Autodesk Inventor part; units mm, degrees
ref_plane "YZ Plane" through (0, 0, 0) normal (1, 0, 0) x (0, 1, 0)
ref_plane "XZ Plane" through (0, 0, 0) normal (0, 1, 0) x (-1, 0, 0)
ref_plane "XY Plane" through (0, 0, 0) normal (0, 0, 1) x (1, 0, 0)
sketch "Boceto1" plane through (0, 0, 0) normal (0, 0, 1) x (1, 0, 0)
  line L0 (85, 15) -> (-82, 15)
  line L1 (-85, -15) -> (85, 15) construction
  line L2 (85, -15) -> (-85, 15) construction
  line L3 (-28, -15) -> (-28, 5)
  line L4 (28, 5) -> (28, -15)
  line L5 (-28, 5) -> (28, 5)
  line L6 (-82, -15) -> (-28, -15)
  line L7 (28, -15) -> (85, -15)
  line L8 (-82, -13.0321) -> (-82, -3.7)
  line L9 (-82, -3.7) -> (-85, -3.7)
  line L10 (-85, -13.0321) -> (-85, -3.7)
  line L11 (-82, -13.0321) -> (-85, -13.0321)
  line L12 (-82, 3.7) -> (-82, 13.0321)
  line L13 (-82, 13.0321) -> (-85, 13.0321)
  line L14 (-85, 3.7) -> (-85, 13.0321)
  line L15 (-82, 3.7) -> (-85, 3.7)
  line L16 (-82, -3.7) -> (-82, 3.7)
  line L17 (-82, 13.0321) -> (-82, 15)
  line L18 (-82, -15) -> (-82, -13.0321)
  line L19 (82, 15) -> (82, 11.3)
  line L20 (82, 11.3) -> (85, 11.3)
  line L21 (85, 15) -> (85, 11.3)
  line L22 (82, 15) -> (85, 15)
  line L23 (82, 3.7) -> (82, -3.7)
  line L24 (82, -3.7) -> (85, -3.7)
  line L25 (85, 3.7) -> (85, -3.7)
  line L26 (82, 3.7) -> (85, 3.7)
  line L27 (82, -11.3) -> (82, -15)
  line L28 (82, -15) -> (85, -15)
  line L29 (85, -11.3) -> (85, -15)
  line L30 (82, -11.3) -> (85, -11.3)
  line L31 (82, -3.7) -> (82, -11.3)
  line L32 (82, 11.3) -> (82, 3.7)
  point P0 (0, 0)
  point P1 (28, 0)
  dimension "d0" = 30
  dimension "d1" = 170
  dimension "d7" = 20
  dimension "d11" = 30
extrude "Extrusión1" add sketch "Boceto1" along normal blind 3
Part model, mm, in its own coordinate system. A direction names the side the tool comes from. Coordinates: 2 decimals unless noted, no trailing zeros. Write each loop counter-clockwise with the first axis right and the second up, starting at its lowest first coordinate (ties: lowest second). Pieces come first, ordered by that corner, then holes.
Item 1: Mould opens along X. For faces 1 (the face through (-85, -8, 1)), 2 (the face through (-83, -3.7, 1)), 3 (the face through (28, -5, 1)) say: released by +X, released by -X, zero draft, split by the parting line, or undercut.
Item 2: Slice it at A-A (y = -2). Write the cut outline in (x, z).
Item 3: Probe line 1 (X direction, y = -0.5, z = 0.35); line 2 (X direction, y = 4.5, z = 0.6); line 3 (Y direction, x = -7, z = 1.75). List the from-to ranges inside material, lowest first.
Item 4: Slice it at C-C (x = 7.5). Write the cut outline in (y, z), and give its area (3 significant figures).
Item 5: Pin check, flat tips, straight feed: pin 1 (0.6 mm diameter, centred on y = 13.5, z = 1, fed in from -X); pin 2 (1.5 mm diameter, centred on x = -83.5, z = 1, fed in from +Y); pin 3 (1.5 mm diameter, centred on y = -5.5, z = 1.5, fed in from +X). Stop position of each tip, or through.
Item 6: Which spindle directions (+Z, -Z, +X, -X, +Y, -Y) get a long thin tool onto all of the face, cutting with end or side? Do faces 4 (the face through (-83, -13.032, 1)), 5 (the face through (0, 5, 1)), 6 (the face through (-83, 3.7, 1)), 7 (the face through (-83, 13.032, 1)), 8 (the face through (83, -11.3, 1)). Say none if no direction does.
Item 7: Slice it at B-B (z = 2.35). Write the cut outline in (x, y), and give its area (3 significant figures).
Results found:
1. face 1: released by -X
1. face 2: zero draft
1. face 3: undercut
2. outline: (-82, 0) - (-28, 0) - (-28, 3) - (-82, 3) - close; (28, 0) - (85, 0) - (85, 3) - (28, 3) - close
3. line 1: x = -82 to -28, 28 to 85
3. line 2: x = -85 to -28, 28 to 82
3. line 3: y = 5 to 15
4. outline: (5, 0) - (15, 0) - (15, 3) - (5, 3) - close
4. area: 30.0 mm2
5. pin 1: stops at x = -82
5. pin 2: stops at y = 13.03
5. pin 3: stops at x = 82
6. face 4: +Z, -Z, -X, -Y
6. face 5: +Z, -Z, -Y
6. face 6: +Z, -Z, -X
6. face 7: +Z, -Z, -X, +Y
6. face 8: +Z, -Z, +X
7. outline: (-85, -13.03) - (-82, -13.03) - (-82, -15) - (-28, -15) - (-28, 5) - (28, 5) - (28, -15) - (85, -15) - (85, -11.3) - (82, -11.3) - (82, -3.7) - (85, -3.7) - (85, 3.7) - (82, 3.7) - (82, 11.3) - (85, 11.3) - (85, 15) - (-82, 15) - (-82, 13.03) - (-85, 13.03) - (-85, 3.7) - (-82, 3.7) - (-82, -3.7) - (-85, -3.7) - close
7. area: 3,900 mm2
